Can you work these out from the model? Positions are in its coordinate system, mm. Face numbers are marked on the shaded views. A direction names the side the tool comes from. Coordinates: 2 decimals unless noted, no trailing zeros. Loops run counter-clockwise (first coordinate to the right, second up) from the corner with the lowest first, then second, coordinate; pieces in that order, holes last. Notation, with made-up numbers: (-10, 5.25) -> (11, 5.25) arc R22 cw to (11, 18.25) -> close; hole circle Ø6 at (82, 2.25). An arc over 180 degrees is marked (long way). Put each result on its own line as item: value. Start each with the question number.
Item 1: Please list where these lines run through material, in increasing order: L1, parallel to X at y = -7, z = 0.35; L2, parallel to Y at x = 11, z = 0.2; L3, parallel to X at y = 2, z = 1.6. Write a range as from..to.
Item 2: If we section it at D-D on y = 2.25: Please give me the cut outline in (x, z).
Item 3: If we section it at A-A on y = -9: Please give me the cut outline in (x, z), plus the area to 3 significant figures.
Item 4: Will these pins go through, and if not, where does the flat tip stop? P1, Ø1.5, axis at x = -5, z = 1.5, coming from the +Y side; P2, Ø1.5, axis at x = 10, z = 1, coming from the -Y side; P3, Ø1.5, axis at y = -8.5, z = 2, coming from the -X side.
Item 5: For the marked faces 1, 2, 3, 4 and 5, which set-ups out of +Z, -Z, +X, -X, +Y, -Y let a thin tool reach every point of the face, with its end or its side?
Item 6: If we section it at B-B on z = 1: Please give me the cut outline in (x, y), plus the area to 3 significant figures.
Item 7: If we section it at C-C on x = 0: Please give me the cut outline in (y, z).
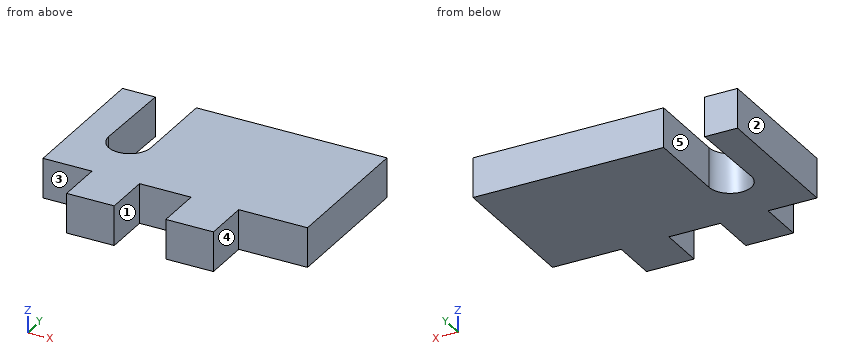
```python
from build123d import *

# Parameters (mm, degrees)
SKETCH1_W           = 20
SKETCH1_H           = 14.5
BOSS_EXTRUDE1_DEPTH = 3
SKETCH2_W           = 3.7
SKETCH2_H           = 3.5
SKETCH2_W_2         = 3.9
SKETCH2_W_3         = 5.2
CUT_EXTRUDE1_DEPTH  = 3
CUT_EXTRUDE2_DEPTH  = 3
CUT_EXTRUDE3_DEPTH  = 3


with BuildPart() as part:
    # Sketch1 → Boss-Extrude1 (new body)
    with BuildSketch(Plane.XY):
        with Locations((2.116182573, -2.915975104)):
            Rectangle(SKETCH1_W, SKETCH1_H)
    extrude(amount=BOSS_EXTRUDE1_DEPTH)

    # Sketch2 → Cut-Extrude1 (cut)
    with BuildSketch(Plane.XY.offset(3)):
        with Locations((-6.033817427, -8.415975104)):
            Rectangle(SKETCH2_W, SKETCH2_H)
        with Locations((1.366182573, -8.415975104)):
            Rectangle(SKETCH2_W_2, SKETCH2_H)
        with Locations((9.516182573, -8.415975104)):
            Rectangle(SKETCH2_W_3, SKETCH2_H)
    extrude(amount=-CUT_EXTRUDE1_DEPTH, mode=Mode.SUBTRACT)

    # Sketch3 → Cut-Extrude2 (cut)
    with BuildSketch(Plane.XY.offset(3)):
        with BuildLine():
            Line((-2.300101836, 4.334024896), (-2.300101836, -1.938179145))
            ThreePointArc((-2.300101836, -1.938179145), (-3.850101836, -3.488179145), (-5.400101836, -1.938179145))
            Line((-5.400101836, -1.938179145), (-5.400101836, 4.334024896))
            ThreePointArc((-5.400101836, 4.334024896), (-3.850101836, 5.884024896), (-2.300101836, 4.334024896))
        make_face()
    extrude(amount=-CUT_EXTRUDE2_DEPTH, mode=Mode.SUBTRACT)

    # Sketch4 → Cut-Extrude3 (cut)
    with BuildSketch(Plane.XY.offset(3)):
        with BuildLine():
            Line((-5.400101836, 4.334024896), (-5.500101836, -1.945141671))
            ThreePointArc((-5.500101836, -1.945141671), (-3.896620573, -3.541660408), (-2.300101836, -1.938179145))
            Line((-2.300101836, -1.938179145), (-5.400101836, 4.334024896))
        make_face()
    extrude(amount=-CUT_EXTRUDE3_DEPTH, mode=Mode.SUBTRACT)


solid = part.part
```
Solutions:
1. L1: -4.18..-0.58, 3.32..6.92
1. L2: -6.67..4.33
1. L3: -7.88..-5.44, -2.3..12.12
2. outline: (-7.88, 0) -> (-5.43, 0) -> (-5.43, 3) -> (-7.88, 3) -> close; (-2.3, 0) -> (12.12, 0) -> (12.12, 3) -> (-2.3, 3) -> close
3. outline: (-4.18, 0) -> (-0.58, 0) -> (-0.58, 3) -> (-4.18, 3) -> close; (3.32, 0) -> (6.92, 0) -> (6.92, 3) -> (3.32, 3) -> close
3. area: 21.6 mm^2
4. P1: y = 4.33
4. P2: y = -6.67
4. P3: x = -4.18
5. face 1: +Z, -Z, -Y
5. face 2: +Z, -Z, -X, +Y, -Y
5. face 3: +Z, -Z, -X, -Y
5. face 4: +Z, -Z, +X, -Y
5. face 5: +Z, -Z, +Y
6. outline: (-7.88, -6.67) -> (-4.18, -6.67) -> (-4.18, -10.17) -> (-0.58, -10.17) -> (-0.58, -6.67) -> (3.32, -6.67) -> (3.32, -10.17) -> (6.92, -10.17) -> (6.92, -6.67) -> (12.12, -6.67) -> (12.12, 4.33) -> (-2.3, 4.33) -> (-2.3, -1.94) arc R1.6 cw to (-5.5, -1.95) -> (-5.4, 4.33) -> (-7.88, 4.33) -> close
6. area: 221 mm^2
7. outline: (-6.67, 0) -> (4.33, 0) -> (4.33, 3) -> (-6.67, 3) -> close
